```python
from build123d import *

# Parameters (mm, degrees)
F3_DEPTH              = 14
F5_DEPTH              = 20
F5_COPIES_COUNT       = 4
F8_D                  = 6
F8_DEPTH              = 3
F8_TIP                = 1.8025818571
F8_ON_F6_D            = 6
F8_ON_F6_DEPTH        = 3
F8_ON_F6_TIP          = 1.8025818571
F8_COPIES_COUNT       = 4
F8_ON_F6_COPIES_COUNT = 4
F9_R                  = 3


# Not quite as in the source:
# - a pattern or mirror of a feature is missing from the dataset's text; its kind, count and spacing are read off the source's solid


with BuildPart() as f3:
    # F2 (on Top) → F3 (new body)
    with BuildSketch(Plane.XY):
        Polygon((-13, 38), (-13, 13), (-38, 13), (-38, -13), (-13, -13), (-13, -38), (13, -38), (13, -13), (38, -13), (38, 13), (13, 13), (13, 38), align=None)
    extrude(amount=-F3_DEPTH)

    # F4 (on Top) → F5 (join)
    with BuildSketch(Plane.XY):
        Polygon((13, 38), (10, 38), (10, 10), (38, 10), (38, 13), (13, 13), align=None)
    f5 = extrude(amount=F5_DEPTH)

    # F5_copies: F5 ×4 about axis
    f5_copies_axis = Axis((0, 0, 0), (0, 0, 1))
    for i in range(1, F5_COPIES_COUNT):
        add(f5.rotate(f5_copies_axis, i * 360 / F5_COPIES_COUNT))

    # F8
    with Locations(Plane.YZ.offset(13)):
        with Locations((27, 12.5)):
            f8 = Hole(F8_D / 2, depth=F8_DEPTH)
            with Locations((0, 0, -(F8_DEPTH + F8_TIP / 2))):  # 118° drill point
                Cone(0, F8_D / 2, F8_TIP, mode=Mode.SUBTRACT)

    # F8 on F6
    with Locations(Plane(origin=(0, 13, 0), x_dir=(-1, 0, 0), z_dir=(0, 1, 0))):
        with Locations((-27, 12.5)):
            f8_on_f6 = Hole(F8_ON_F6_D / 2, depth=F8_ON_F6_DEPTH)
            with Locations((0, 0, -(F8_ON_F6_DEPTH + F8_ON_F6_TIP / 2))):  # 118° drill point
                Cone(0, F8_ON_F6_D / 2, F8_ON_F6_TIP, mode=Mode.SUBTRACT)

    # F8_copies: F8 ×4 about axis
    f8_copies_axis = Axis((0, 0, 0), (0, 0, 1))
    for i in range(1, F8_COPIES_COUNT):
        add(f8.rotate(f8_copies_axis, i * 360 / F8_COPIES_COUNT), mode=Mode.SUBTRACT)

    # F8 on F6_copies: F8 on F6 ×4 about axis
    f8_on_f6_copies_axis = Axis((0, 0, 0), (0, 0, 1))
    for i in range(1, F8_ON_F6_COPIES_COUNT):
        add(f8_on_f6.rotate(f8_on_f6_copies_axis, i * 360 / F8_ON_F6_COPIES_COUNT), mode=Mode.SUBTRACT)

    # F9
    f9_edges = [f3.edges().sort_by_distance(p)[0] for p in [
        (10, 10, 10),
        (-10, 10, 10),
        (-10, -10, 10),
        (10, -10, 10),
    ]]
    fillet(f9_edges, radius=F9_R)


solid = f3.part
```
Here's how the part is built. I have some questions about the finished solid (model axes, mm). A direction names the side the tool comes from. Give positions to 0.01 mm unless a question says otherwise; leave off trailing zeros. Write each loop counter-clockwise with the first axis right and the second up, starting at its lowest first coordinate (ties: lowest second). Pieces come first, ordered by that corner, then holes. Notation, with made-up numbers: (89.25, -2.75) -> (112.25, -2.75) arc R17 cw to (112.25, 18.25) -> close; hole circle Ø4 at (77, 54). An arc over 180 degrees is marked (long way). Write each question's results on one line, items separated by ' | '.
Item 1: Suppose I cut it at C-C on z = 5.5. Write out the boundary of the cut face in (x, y).
Output:
outline: (-38, -13) -> (-13, -13) -> (-13, -38) -> (-10, -38) -> (-10, -13) arc R3 ccw to (-13, -10) -> (-38, -10) -> close; (-38, 10) -> (-13, 10) arc R3 ccw to (-10, 13) -> (-10, 38) -> (-13, 38) -> (-13, 13) -> (-38, 13) -> close; (10, -38) -> (13, -38) -> (13, -13) -> (38, -13) -> (38, -10) -> (13, -10) arc R3 ccw to (10, -13) -> close; (10, 13) arc R3 ccw to (13, 10) -> (38, 10) -> (38, 13) -> (13, 13) -> (13, 38) -> (10, 38) -> close
Item 2: Suppose I cut it at A-A on x = 27. Write out the boundary of the cut face in (y, z).
Output:
outline: (-13, -14) -> (13, -14) -> (13, 9.5) -> (10, 9.5) -> (10, 0) -> (-10, 0) -> (-10, 9.5) -> (-13, 9.5) -> close; (-13, 15.5) -> (-10, 15.5) -> (-10, 20) -> (-13, 20) -> close; (10, 15.5) -> (13, 15.5) -> (13, 20) -> (10, 20) -> close
Item 3: Suppose I cut it at D-D on y = -32. Write out the boundary of the cut face in (x, z).
Output:
outline: (-13, -14) -> (13, -14) -> (13, 20) -> (10, 20) -> (10, 0) -> (-10, 0) -> (-10, 20) -> (-13, 20) -> close
Item 4: On a 3-axis mill with a long thin cutter (end or side, diameter ignored), from which of +Z, -Z, +X, -X, +Y, -Y can I reach the whole of each face in a straight line? I mean faces 1 (the face through (-26, -13, 3)), 2 (the face through (-10, 25, 10)), 3 (the face through (-10.86, -10.9, 10.14)), 4 (the face through (26, -10, 8)). Say none if no direction works.
Output:
face 1: +Z, -Z, -X, -Y | face 2: +Z, +Y, -Y | face 3: +Z | face 4: +Z, +X, -X
Item 5: We'd pull the mould along X, two halves only. Please class faces 5 (the face through (-1, 1, -14)), 6 (the face through (10.9, -10.86, 10.14)), 7 (the face through (-10.9, 10.86, 10.14)), 8 (the face through (-13, -25, 3)): pulls with the +X half, pulls with the -X half, needs draft (parallel to the pull), parting line crosses it, or undercut.
Output:
face 5: needs draft | face 6: undercut | face 7: undercut | face 8: pulls with the -X half
Item 6: If I drill on L1, parallel to X at y = -14.5, z = 15; L2, parallel to Y at x = -11.5, z = 10, over which ranges is the centre line in solid material (lowest first)?
Output:
L1: x = -13 to -10, 10 to 13 | L2: y = -38 to -28.66, -25.34 to -10.4, 10.4 to 25.34, 28.66 to 38
Item 7: For pin 1 Ø1 at (y, z) = (-19, -5.5) entering from -X; pin 2 Ø8 at (x, z) = (-27, 12.5) entering from +Y; pin 3 Ø7.5 at (x, z) = (-28, -2.5) entering from -Y; pin 4 Ø12 at (x, y) = (30.5, 20.5) entering from +Z, each with a flat end and sliding along its axis, tell me the tip position at first contact or that it passes through.
Output:
pin 1: stops at x = -13 | pin 2: stops at y = 13 | pin 3: stops at y = -13 | pin 4: passes through
